Check sheet for the drawn part. Datum: minimum x, y, z corner. Units: mm. A direction names the side the tool comes from. Coordinates: 2 decimals unless noted, no trailing zeros. Write each loop counter-clockwise with the first axis right and the second up, starting at its lowest first coordinate (ties: lowest second). Pieces come first, ordered by that corner, then holes. Notation, with made-up numbers: (17, 76.25) -> (37, 76.25) arc R21 cw to (37, 87.25) -> close; hole circle Ø5 at (-12, 77). An arc over 180 degrees is marked (long way). Answer in a Markdown table with one row per item.
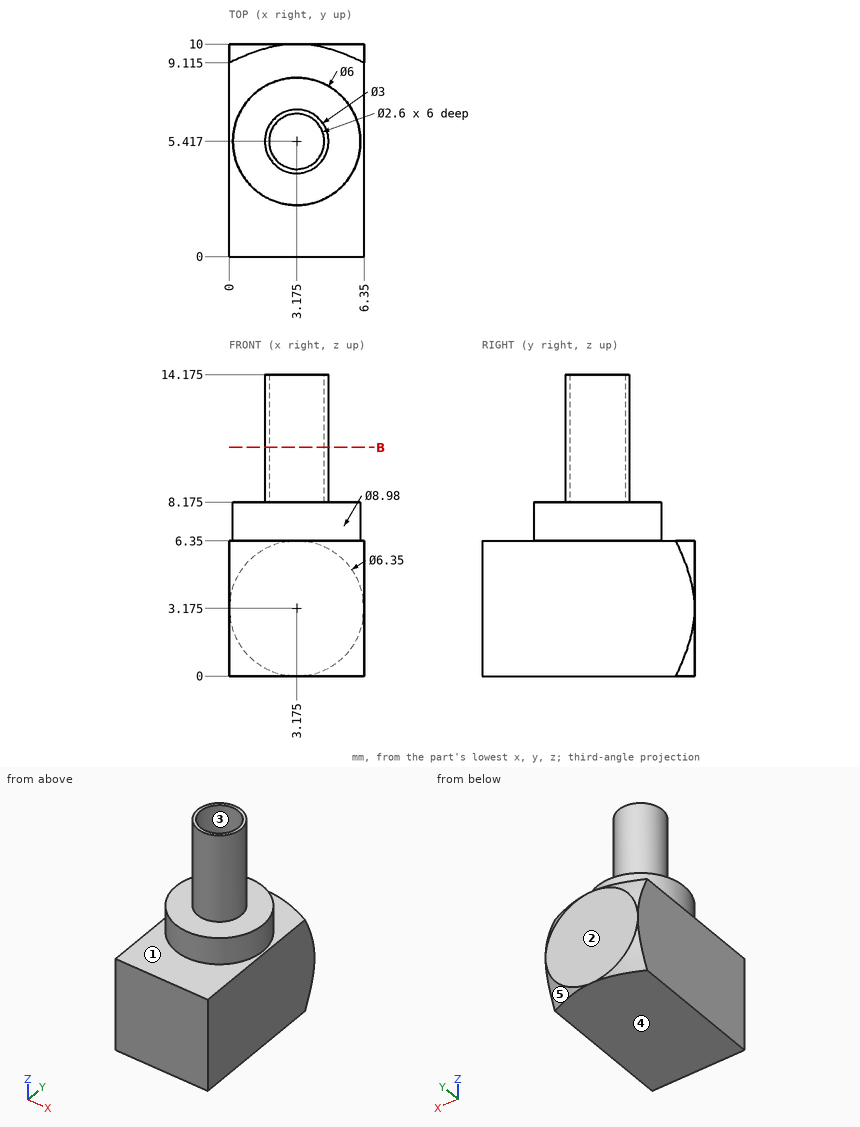
1. Sectioned sample at B-B, the plane z = 10.75. Record the cut outline in (x, y) (1 decimal).
Findings below:
| item | result |
|---|---|
| outline | circle Ø3 at (3.2, 5.4); hole circle Ø2.6 at (3.2, 5.4) |
2. Access from +Z, -Z, +X, -X, +Y, -Y to the whole of each face (thin tool, end or side, straight path). Record for the marked faces 1 and 2.
Findings below:
| item | result |
|---|---|
| face 1 | +Z |
| face 2 | +Z, -Z, +X, -X, +Y |
3. Release check for a two-part mould opening along X. For the marked faces 3, 4 and 5 record: released by +X, released by -X, zero draft, split by the parting line, or undercut.
Findings below:
| item | result |
|---|---|
| face 3 | undercut |
| face 4 | zero draft |
| face 5 | released by +X |
4. Go/stop test with flat-tipped pins: pin 1 (0.8 mm diameter, centred on x = 3, y = 5.5, fed in from +Z) (3 decimals); pin 2 (1 mm diameter, centred on x = 5, z = 12, fed in from +Y); pin 3 (5 mm diameter, centred on y = 2.5, z = 11, fed in from -X). Record where each tip stops, or that it passes through.
Findings below:
| item | result |
|---|---|
| pin 1 | stops at z = 8.175 |
| pin 2 | stops at y = 6.12 |
| pin 3 | stops at x = 1.73 |
5. Material ranges on probe 1 along Z at (x, y) = (5.75, 3); probe 2 along Y at (x, z) = (3.25, 10.75) (1 decimal); probe 3 along Z at (x, y) = (2.25, 5.5) (1 decimal), recorded low to high. Write a range as from..to.
Findings below:
| item | result |
|---|---|
| probe 1 | z = 0..6.35 |
| probe 2 | y = 3.9..4.1, 6.7..6.9 |
| probe 3 | z = 0..8.2 |
